Geometry: final body of the model. Coordinates: model frame, mm. A direction names the side the tool comes from. Coordinates: 2 decimals unless noted, no trailing zeros. Write each loop counter-clockwise with the first axis right and the second up, starting at its lowest first coordinate (ties: lowest second). Pieces come first, ordered by that corner, then holes. Notation, with made-up numbers: (-13.75, -35) -> (7.25, -35) arc R33 ccw to (7.25, 1) -> close; hole circle Ø10 at (59.5, 28). An arc over 180 degrees is marked (long way). One line per item, written item: value.
```python
from build123d import *

# Parameters (mm, degrees)
F0_R     = 380.9365
F0_R_2   = 236.5375
F1_DEPTH = 304.8
F6_R     = 1.27
F7_DEPTH = 380.9375


with BuildPart() as f1:
    # F0 (on Front) → F1 (new body)
    with BuildSketch(Plane.XZ):
        Circle(F0_R)
        Circle(F0_R_2, mode=Mode.SUBTRACT)
    extrude(amount=-F1_DEPTH)

    # F2 (on Right) → F3 (revolve, cut)
    with BuildSketch(Plane.YZ):
        Polygon((-0.674657, 0), (0, 0), (9.525, 0), (9.525, 323.444068), (0, 325.9074), (-38.13795, 325.9074), align=None)
    revolve(axis=Axis((0, -111.905819, 0), (0, -1, 0)), mode=Mode.SUBTRACT)

    # F4 (on Right) → F5 (revolve, cut)
    with BuildSketch(Plane.YZ):
        Polygon((39.294728, 254.3556), (9.525, 266.9921), (-83.954796, 266.9921), (-48.076838, 187.997639), (83.789648, 229.984577), (72.7964, 240.977825), (52.705, 252.5776), (45.438306, 252.5776), (41.2496, 254.3556), align=None)
    revolve(axis=Axis((0, 0, 0), (0, -1, 0)), mode=Mode.SUBTRACT)

    # F6 (on Top) → F7 (cut, through all)
    with BuildSketch(Plane.XY):
        with Locations((0, 65.6082)):
            Circle(F6_R)
    extrude(amount=F7_DEPTH, mode=Mode.SUBTRACT)


solid = f1.part
```
(1) Pull-direction query (Z, two-part tool) for faces 1 (the cylindrical face through (-49.59, 150.266, 377.695)), 2 (the flat face through (280, 0, 171)), 3 (the conical face through (226.36, 37.43, 117.73)); classes: released by +Z, released by -Z, zero draft, split by the parting line, or undercut.
Responses:
face 1: split by the parting line
face 2: zero draft
face 3: undercut
(2) Section B-B (y = 273). Return the cut outline in (x, z) (1 decimal), then the cut area to 3 significant figures.
Responses:
outline: circle Ø761.9 at (0, 0); hole circle Ø473.1 at (0, 0)
area: 280,000 mm2
(3) First-contact query: pin 1 (12 mm diameter, centred on x = 169.5, y = 130, fed in from -Z); pin 2 (3 mm diameter, centred on y = 91.5, z = 214.5, fed in from +X); pin 3 (12 mm diameter, centred on y = 44.5, z = 123, fed in from +X). Flat tips, straight axial feed; report the tip coordinate or a pass-through.
Responses:
pin 1: stops at z = -344.06
pin 2: stops at x = 315.82
pin 3: stops at x = 362.52
(4) Line query: line 1 (Y direction, x = 0, z = 297) (3 decimals); line 2 (Z direction, x = -8, y = 269); line 3 (Z direction, x = 0, y = 50). Output: solid intervals per line, ascending. Write a range as [from, to].
Responses:
line 1: y = [9.525, 64.338], [66.878, 304.8]
line 2: z = [-380.85, -236.4], [236.4, 380.85]
line 3: z = [-380.94, -252.58], [252.58, 380.94]
(5) Section A-A (z = 0). Return the cut outline in (x, y) (1 decimal).
Responses:
outline: (-380.9, 0) -> (-325.9, 0) -> (-323.4, 9.5) -> (-267, 9.5) -> (-254.4, 39.3) -> (-254.4, 41.2) -> (-252.6, 45.4) -> (-252.6, 52.7) -> (-241, 72.8) -> (-236.5, 77.2) -> (-236.5, 304.8) -> (-380.9, 304.8) -> close; (236.5, 77.2) -> (241, 72.8) -> (252.6, 52.7) -> (252.6, 45.4) -> (254.4, 41.2) -> (254.4, 39.3) -> (267, 9.5) -> (323.4, 9.5) -> (325.9, 0) -> (380.9, 0) -> (380.9, 304.8) -> (236.5, 304.8) -> close
(6) Reachability of faces 4 (the cylindrical face through (109.15, 189.43, -209.85)), 5 (the cylindrical face through (246.571, 49.021, -54.754)) from +Z, -Z, +X, -X, +Y, -Y: full face, straight path, thin tool, end or side. Return the list, or none.
Responses:
face 4: +Y, -Y
face 5: -Y
